```python
from build123d import *

# Parameters (mm, degrees)
F1_DEPTH = 3.175


with BuildPart() as f1:
    # F0 (on Front) → F1 (new body)
    with BuildSketch(Plane.XZ):
        with BuildLine():
            ThreePointArc((0, 7.62), (-5.599533552, 5.1681354471), (-7.5955768603, -0.6096))
            ThreePointArc((-7.5955768603, -0.6096), (0.3050445253, -7.6138917669), (7.62, 0))
            ThreePointArc((7.62, 0), (5.3881536726, 5.3881536726), (0, 7.62))
        make_face()
        with BuildLine():
            ThreePointArc((3.175, 0), (-2.2450640303, -2.2450640303), (0, 3.175))
            ThreePointArc((0, 3.175), (2.2450640303, 2.2450640303), (3.175, 0))
        make_face(mode=Mode.SUBTRACT)
        with BuildLine():
            Line((-11.140179395, 43.55592), (-7.5955768603, -0.6096))
            ThreePointArc((-7.5955768603, -0.6096), (-5.599533552, 5.1681354471), (0, 7.62))
            Line((0, 7.62), (0, 33.274))
            ThreePointArc((0, 33.274), (-7.5799319891, 36.2373507904), (-11.140179395, 43.55592))
        make_face()
        with BuildLine():
            Line((62.366144, 60.1571281452), (-0.804672, 55.5969941676))
            ThreePointArc((-0.804672, 55.5969941676), (7.612816881, 52.6321754525), (11.176, 44.45))
            Line((11.176, 44.45), (47.752, 44.45))
            ThreePointArc((47.752, 44.45), (51.9705709533, 55.1771510596), (62.366144, 60.1571281452))
        make_face()
        with BuildLine():
            ThreePointArc((79.248, 44.45), (75.1524558974, 33.8566164253), (64.99606, 28.7732239132))
            Line((64.99606, 28.7732239132), (115.33759, 33.5773972301))
            ThreePointArc((115.33759, 33.5773972301), (106.9529759079, 36.3684580067), (103.378, 44.45))
            Line((103.378, 44.45), (100.0252, 44.45))
            Line((100.0252, 44.45), (79.248, 44.45))
        make_face()
        with BuildLine():
            ThreePointArc((125.222, 44.45), (122.3815419933, 51.7970240921), (115.33759, 55.3226027699))
            ThreePointArc((115.33759, 55.3226027699), (106.9529759079, 52.5315419933), (103.378, 44.45))
            ThreePointArc((103.378, 44.45), (106.9529759079, 36.3684580067), (115.33759, 33.5773972301))
            ThreePointArc((115.33759, 33.5773972301), (122.3815419933, 37.1029759079), (125.222, 44.45))
        make_face()
        with BuildLine():
            ThreePointArc((117.475, 44.45), (114.3, 41.275), (111.125, 44.45))
            ThreePointArc((111.125, 44.45), (114.3, 47.625), (117.475, 44.45))
        make_face(mode=Mode.SUBTRACT)
        with BuildLine():
            ThreePointArc((-0.804672, 55.5969941676), (-8.4803735466, 51.7291648223), (-11.140179395, 43.55592))
            ThreePointArc((-11.140179395, 43.55592), (-7.5799319891, 36.2373507904), (0, 33.274))
            Line((0, 33.274), (0, 41.275))
            ThreePointArc((0, 41.275), (-2.2450640303, 46.6950640303), (3.175, 44.45))
            Line((3.175, 44.45), (11.176, 44.45))
            ThreePointArc((11.176, 44.45), (7.612816881, 52.6321754525), (-0.804672, 55.5969941676))
        make_face()
        with BuildLine():
            ThreePointArc((64.99606, 60.1267760868), (63.6817367499, 60.1969513162), (62.366144, 60.1571281452))
            ThreePointArc((62.366144, 60.1571281452), (51.9705709533, 55.1771510596), (47.752, 44.45))
            Line((47.752, 44.45), (60.325, 44.45))
            ThreePointArc((60.325, 44.45), (63.5, 47.625), (66.675, 44.45))
            Line((66.675, 44.45), (79.248, 44.45))
            ThreePointArc((79.248, 44.45), (75.1524558974, 55.0433835747), (64.99606, 60.1267760868))
        make_face()
        with BuildLine():
            ThreePointArc((47.752, 44.45), (51.970558664, 33.7228621488), (62.3661080111, 28.7428744527))
            ThreePointArc((62.3661080111, 28.7428744527), (63.6817187098, 28.7030484756), (64.99606, 28.7732239132))
            ThreePointArc((64.99606, 28.7732239132), (75.1524558974, 33.8566164253), (79.248, 44.45))
            Line((79.248, 44.45), (66.675, 44.45))
            ThreePointArc((66.675, 44.45), (63.5, 41.275), (60.325, 44.45))
            Line((60.325, 44.45), (47.752, 44.45))
        make_face()
        with BuildLine():
            Line((115.33759, 55.3226027699), (64.99606, 60.1267760868))
            ThreePointArc((64.99606, 60.1267760868), (75.1524558974, 55.0433835747), (79.248, 44.45))
            Line((79.248, 44.45), (100.0252, 44.45))
            Line((100.0252, 44.45), (103.378, 44.45))
            ThreePointArc((103.378, 44.45), (106.9529759079, 52.5315419933), (115.33759, 55.3226027699))
        make_face()
        with BuildLine():
            ThreePointArc((103.2002, 47.625), (102.2702640303, 45.3799359697), (100.0252, 44.45))
            ThreePointArc((100.0252, 44.45), (97.7801359697, 49.8700640303), (103.2002, 47.625))
        make_face(mode=Mode.SUBTRACT)
        with BuildLine():
            Line((0, 41.275), (0, 33.274))
            ThreePointArc((0, 33.274), (7.9026253865, 36.5473746135), (11.176, 44.45))
            Line((11.176, 44.45), (3.175, 44.45))
            ThreePointArc((3.175, 44.45), (2.2450640303, 42.2049359697), (0, 41.275))
        make_face()
        with BuildLine():
            ThreePointArc((0, 7.62), (5.3881536726, 5.3881536726), (7.62, 0))
            Line((7.62, 0), (9.5838374982, 24.7157604221))
            ThreePointArc((9.5838374982, 24.7157604221), (12.3022276898, 30.0648572861), (18.000044724, 31.9456452964))
            Line((18.000044724, 31.9456452964), (62.3661080111, 28.7428744527))
            ThreePointArc((62.3661080111, 28.7428744527), (51.970558664, 33.7228621488), (47.752, 44.45))
            Line((47.752, 44.45), (11.176, 44.45))
            ThreePointArc((11.176, 44.45), (7.9026253865, 36.5473746135), (0, 33.274))
            Line((0, 33.274), (0, 7.62))
        make_face()
    extrude(amount=F1_DEPTH)


solid = f1.part
```
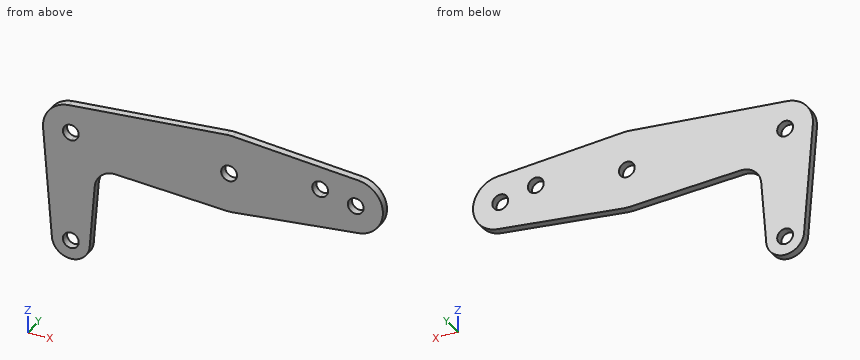
Input: part model. Units: mm. Frame: model coordinates. Round coordinates to 2 decimals unless told otherwise and drop trailing zeros. Loops run counter-clockwise (first coordinate to the right, second up) from the corner with the lowest first, then second, coordinate; pieces in that order, holes last. Notation, with made-up numbers: (72, -30) -> (126, -30) arc R27 ccw to (126, -12) -> close; hole circle Ø8 at (-23.75, 76). An arc over 180 degrees is marked (long way). Write each question's results on one line, items separated by ' | '.
1. Section B-B (z = 26.5). Return loops of the section in (x, y) (3 decimals), and give its area (3 significant figures).
Geometry results:
outline: (-9.771, -3.175) -> (9.936, -3.175) -> (9.936, 0) -> (-9.771, 0) -> close | area: 62.6 mm2
2. Section A-A (y = -1.5). Return loops of the section in (x, z) (3 decimals).
Geometry results:
outline: (-11.14, 43.556) -> (-7.596, -0.61) arc R7.62 ccw to (7.62, 0) -> (9.584, 24.716) arc R7.874 cw to (18, 31.946) -> (62.366, 28.743) arc R15.748 ccw to (64.996, 28.773) -> (115.338, 33.577) arc R10.922 ccw to (115.338, 55.323) -> (64.996, 60.127) arc R15.748 ccw to (62.366, 60.157) -> (-0.805, 55.597) arc R11.176 ccw to start; hole circle Ø6.35 at (0, 0); hole circle Ø6.35 at (0, 44.45); hole circle Ø6.35 at (63.5, 44.45); hole circle Ø6.35 at (100.025, 47.625); hole circle Ø6.35 at (114.3, 44.45)
3. Section C-C (x = 74.5). Return loops of the section in (y, z) (3 decimals).
Geometry results:
outline: (-3.175, 29.68) -> (0, 29.68) -> (0, 59.22) -> (-3.175, 59.22) -> close
4. Ray query, line 1 (Z direction, x = 0, y = -2.45) (3 decimals); line 2 (Z direction, x = 63.5, y = -1.15) (3 decimals); line 3 (X direction, y = -1.2, z = 45). Return the intervals inside material, ascending. Write a range as from..to.
Geometry results:
line 1: -7.62..-3.175, 3.175..41.275, 47.625..55.655 | line 2: 28.702..41.275, 47.625..60.198 | line 3: -11.16..-3.13, 3.13..60.37, 66.63..98.24, 101.81..111.17, 117.43..125.21
5. First-contact query: P1, Ø4, axis at x = 0, z = 0, coming from the +Y side. Flat tip, straight axial feed; report the tip coordinate or a pass-through.
Geometry results:
P1: through
